from build123d import *

# Parameters (mm, degrees)
BOSS_EXTRUDE1_DEPTH              = 20
CUT_EXTRUDE1_START               = -4
SKETCH2_R                        = 1.625
CUT_EXTRUDE1_DEPTH               = 25
BOSS_EXTRUDE2_DEPTH              = 36.8
CUT_EXTRUDE2_DEPTH               = 45
CUT_EXTRUDE3_REACH               = 43.8
CUT_EXTRUDE3_OFFSET_FROM_SURFACE = 5
SKETCH6_R                        = 3
CUT_EXTRUDE4_DEPTH               = 19


with BuildPart() as part:
    # Sketch1 → Boss-Extrude1 (new body)
    with BuildSketch(Plane(origin=(0, 0, 0), x_dir=(1, 0, 0), z_dir=(0, 1, 0))):
        Polygon((0, 0), (18.4, 0), (18.4, 20), (31.8, 20), (31.8, 23), (13.4, 23), (13.4, 3), (0, 3), align=None)
    extrude(amount=BOSS_EXTRUDE1_DEPTH)

    # Sketch2 → Cut-Extrude1 (cut)
    with BuildSketch(Plane.XY.offset(-20).offset(CUT_EXTRUDE1_START)):
        with Locations((25.1, 2.8)):
            Circle(SKETCH2_R)
        with Locations((25.1, 17.5)):
            Circle(SKETCH2_R)
    cut_extrude1 = extrude(amount=CUT_EXTRUDE1_DEPTH, mode=Mode.SUBTRACT)

    # Mirror1: Cut-Extrude1 across plane
    add(cut_extrude1.mirror(Plane.ZY.offset(-15.9)), mode=Mode.SUBTRACT)

    # Sketch3 → Boss-Extrude2 (add)
    with BuildSketch(Plane.ZY):
        Polygon((0, 0), (0, -24), (18, -24), (14, 8), (14, 20), (0, 20), align=None)
        with BuildLine():
            Line((10.55, -9), (10.55, -19))
            ThreePointArc((10.55, -19), (8, -21.55), (5.45, -19))
            Line((5.45, -19), (5.45, -9))
            ThreePointArc((5.45, -9), (8, -6.45), (10.55, -9))
        make_face(mode=Mode.SUBTRACT)
    extrude(amount=-BOSS_EXTRUDE2_DEPTH)

    # Sketch4 → Cut-Extrude2 (cut, through all)
    with BuildSketch(Plane.XZ.offset(24)):
        Polygon((36.8, 18), (36.416667761, 0), (36.8, 0), align=None)
    extrude(amount=-CUT_EXTRUDE2_DEPTH, mode=Mode.SUBTRACT)

    # Cut-Extrude3: up to this face of the body (flat: up to its plane, moved by the offset)
    cut_extrude3_end = Plane(part.part.faces().sort_by_distance((36.581905222, -1.783418912, 7.75899858))[0]).offset(-CUT_EXTRUDE3_OFFSET_FROM_SURFACE)
    # Sketch5 → Cut-Extrude3 (cut, up to the picked face)
    with BuildSketch(Plane.ZY, mode=Mode.PRIVATE) as cut_extrude3_sk1:
        with BuildLine():
            Line((14, -9), (14, -24))
            Line((14, -24), (2, -24))
            Line((2, -24), (2, -9))
            ThreePointArc((2, -9), (8, -3), (14, -9))
        make_face()
    cut_extrude3_tool1 = split(extrude(cut_extrude3_sk1.sketch, amount=-CUT_EXTRUDE3_REACH, mode=Mode.PRIVATE), bisect_by=cut_extrude3_end, keep=Keep.BOTH, mode=Mode.PRIVATE)
    add(cut_extrude3_tool1.solids().sort_by_distance((0, -14.098317, 8))[0], mode=Mode.SUBTRACT)

    # Sketch6 → Cut-Extrude4 (cut, through all)
    with BuildSketch(Plane(origin=(0, 0, 0), x_dir=(-1, 0, 0), z_dir=(0, 0, -1))):
        with Locations((-6.7, 2.8)):
            Circle(SKETCH6_R)
        with Locations((-6.7, 17.5)):
            Circle(SKETCH6_R)
    extrude(amount=-CUT_EXTRUDE4_DEPTH, mode=Mode.SUBTRACT)


solid = part.part
Can you work these out from the model? Positions are in its coordinate system, mm. A direction names the side the tool comes from. Coordinates: 2 decimals unless noted, no trailing zeros. Loops run counter-clockwise (first coordinate to the right, second up) from the corner with the lowest first, then second, coordinate; pieces in that order, holes last. Notation, with made-up numbers: M -37,-18 L 13,-18 A21 ccw 13,-3 Z; hole C -37,21.25 d8. An arc over 180 degrees is marked long. Answer as CSV lines item,"result". Start each with the question number.
1. For faces 5 (the face through (24.748, 15.914, -21.521)), 6 (the face through (18.4, 10, -10)), 7 (the face through (7, 10, -3)), which set-ups out of +Z, -Z, +X, -X, +Y, -Y let a thin tool reach every point of the face, with its end or its side?
2. Suppose I cut it at C-C, the plane x = 29. List the corners of the cut face in (y, z) for me, plus the area to 3 significant figures.
3. Thinking about a two-plate mould opening in Z: for faces 1 (the face through (5, 2, 0)), 2 (the face through (13.4, 10, -13)), 3 (the face through (34.05, -21.55, 8.06)), 4 (the face through (16, -3, 8)), which applies, +Z half, -Z half, draft (parallel to the pull), parting line (faces both ways), or undercut?
4. Suppose I cut it at B-B, the plane x = 25.1. List the corners of the cut face in (y, z) for me (3 decimals).
5. Suppose I cut it at D-D, the plane z = 8. List the corners of the cut face in (x, y) for me, plus the area to 3 significant figures.
6. Suppose I cut it at A-A, the plane y = 17.5. List the corners of the cut face in (x, z) for me (3 decimals).
7. For pin 1 Ø16 at (y, z) = (12, -5.5) entering from +X; pin 2 Ø6 at (x, z) = (16, -16) entering from -Y; pin 3 Ø4 at (x, y) = (8.5, 14) entering from -Z; pin 4 Ø1.9 at (x, y) = (6.7, 2.8) entering from +Z, each with a flat end and sliding along its axis, tell me the tip position at first contact or that it passes through.
8. If I drill on probe 1 along X at (y, z) = (17.5, -21.9) (3 decimals); probe 2 along Y at (x, z) = (9, 3); probe 3 along Y at (x, z) = (6, -2), over which ranges is the centre line in solid material (lowest first)? Write a range as [from, to].
Output:
1,face 5,"-Z"
1,face 6,"+X, +Y, -Y"
1,face 7,"-Z, -X, +Y, -Y"
2,outline,"M -24,0 L 20,0 L 20,14 L 8,14 L -24,18 L -24,14 L -9,14 A6 cw -9,2 L -24,2 Z; M 0,-23 L 20,-23 L 20,-20 L 0,-20 Z"
2,area,"503 mm^2"
3,face 1,"+Z half"
3,face 2,"draft"
3,face 3,"undercut"
3,face 4,"undercut"
4,outline,"M -24,0 L 20,0 L 20,14 L 8,14 L -24,18 L -24,14 L -9,14 A6 cw -9,2 L -24,2 Z; M 0,-23 L 1.175,-23 L 1.175,-20 L 0,-20 Z; M 4.425,-23 L 15.875,-23 L 15.875,-20 L 4.425,-20 Z; M 19.125,-23 L 20,-23 L 20,-20 L 19.125,-20 Z"
5,outline,"M 0,-3 L 31.59,-3 L 31.59,-6.45 L 36.59,-6.45 L 36.59,20 L 8.36,20 A3 cw long 5.04,20 L 0,20 Z; M 31.59,-24 L 36.59,-24 L 36.59,-21.55 L 31.59,-21.55 Z; hole C 6.7,2.8 d6"
5,area,"816 mm^2"
6,outline,"M 0,-3 L 5.075,-3 L 5.075,0 L 3.7,0 L 3.7,14 L 0,14 Z; M 8.325,-3 L 13.4,-3 L 13.4,-23 L 23.475,-23 L 23.475,-20 L 18.4,-20 L 18.4,0 L 36.417,0 L 36.715,14 L 9.7,14 L 9.7,0 L 8.325,0 Z; M 26.725,-23 L 31.8,-23 L 31.8,-20 L 26.725,-20 Z"
7,pin 1,"stops at x = 36.47"
7,pin 2,"stops at y = 0"
7,pin 3,"stops at z = -3"
7,pin 4,"passes through"
8,probe 1,"x = [13.4, 23.475], [26.725, 31.8]"
8,probe 2,"y = [-5.68, 0.87], [4.73, 15.57], [19.43, 20]"
8,probe 3,"y = [0, 1.33], [4.27, 16.03], [18.97, 20]"
